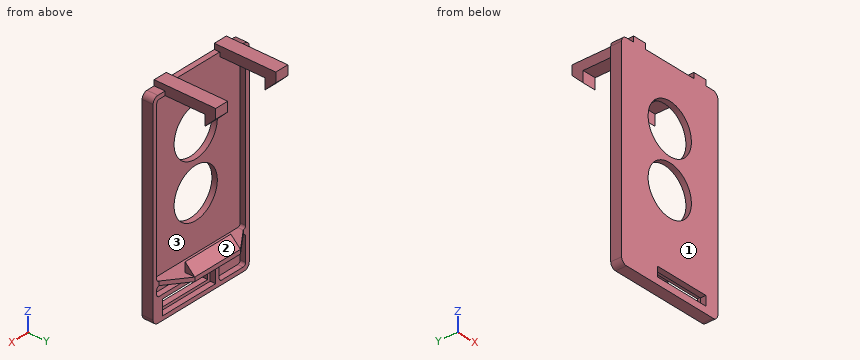
from build123d import *

# Parameters (mm, degrees)
BOSS_EXTRUDE1_DEPTH  = 1
PCB_HOLDER_52_R      = 4.5
BOSS_EXTRUDE2_DEPTH  = 1
BOSS_EXTRUDE3_DEPTH  = 2
PCB_HOLDER_57_W      = 17.5
PCB_HOLDER_57_H      = 0.75
BOSS_EXTRUDE7_DEPTH  = 5
SKETCH6_W            = 9.5
SKETCH6_H            = 1.75
BOSS_EXTRUDE9_DEPTH  = 1.75
CUT_EXTRUDE7_DEPTH   = 0.75
PCB_HOLDER_58_W      = 2.5
PCB_HOLDER_58_H      = 1
PCB_HOLDER_58_H_2    = 0.75
BOSS_EXTRUDE10_DEPTH = 11.25
SKETCH10_W           = 2.5
SKETCH10_H           = 2
BOSS_EXTRUDE11_DEPTH = 2
CUT_EXTRUDE8_DEPTH   = 15
CUT_EXTRUDE12_DEPTH  = 9.5
SKETCH12_W           = 11
SKETCH12_H           = 2.75
SKETCH12_W_2         = 10
SKETCH12_H_2         = 1.75
CUT_EXTRUDE15_DEPTH  = 1
SKETCH12_3_W         = 10
SKETCH12_3_H         = 1.75
CUT_EXTRUDE16_DEPTH  = 2


with BuildPart() as part:
    # PCB holder → Boss-Extrude1 (new body)
    with BuildSketch(Plane(origin=(0, 0, 0), x_dir=(1, 0, 0), z_dir=(0, 1, 0))):
        with BuildLine():
            Line((9, 21.5), (-9, 21.5))
            ThreePointArc((-9, 21.5), (-9.707106781, 21.207106781), (-10, 20.5))
            Line((-10, 20.5), (-10, -14.5))
            ThreePointArc((-10, -14.5), (-9.707106781, -15.207106781), (-9, -15.5))
            Line((-9, -15.5), (9, -15.5))
            ThreePointArc((9, -15.5), (9.707106781, -15.207106781), (10, -14.5))
            Line((10, -14.5), (10, 20.5))
            ThreePointArc((10, 20.5), (9.707106781, 21.207106781), (9, 21.5))
        make_face()
        with BuildLine():
            Line((9.25, 14.25), (9.25, -14.25))
            ThreePointArc((9.25, -14.25), (9.103553391, -14.603553391), (8.75, -14.75))
            Line((8.75, -14.75), (-8.75, -14.75))
            ThreePointArc((-8.75, -14.75), (-9.103553391, -14.603553391), (-9.25, -14.25))
            Line((-9.25, -14.25), (-9.25, 14.25))
            ThreePointArc((-9.25, 14.25), (-9.103553391, 14.603553391), (-8.75, 14.75))
            Line((-8.75, 14.75), (8.75, 14.75))
            ThreePointArc((8.75, 14.75), (9.103553391, 14.603553391), (9.25, 14.25))
        make_face(mode=Mode.SUBTRACT)
    extrude(amount=BOSS_EXTRUDE1_DEPTH)

    # PCB holder<52> → Boss-Extrude2 (add)
    with BuildSketch(Plane(origin=(0, 0, 0), x_dir=(1, 0, 0), z_dir=(0, 1, 0))):
        with BuildLine():
            Line((-9.25, 14.25), (-9.25, -14.25))
            ThreePointArc((-9.25, -14.25), (-9.103553391, -14.603553391), (-8.75, -14.75))
            Line((-8.75, -14.75), (8.75, -14.75))
            ThreePointArc((8.75, -14.75), (9.103553391, -14.603553391), (9.25, -14.25))
            Line((9.25, -14.25), (9.25, 14.25))
            ThreePointArc((9.25, 14.25), (9.103553391, 14.603553391), (8.75, 14.75))
            Line((8.75, 14.75), (-8.75, 14.75))
            ThreePointArc((-8.75, 14.75), (-9.103553391, 14.603553391), (-9.25, 14.25))
        make_face()
        with Locations(Location((0, -5, 0), (0, 0, 270))):
            Circle(PCB_HOLDER_52_R, mode=Mode.SUBTRACT)
        with Locations(Location((0, 5, 0), (0, 0, 270))):
            Circle(PCB_HOLDER_52_R, mode=Mode.SUBTRACT)
    extrude(amount=BOSS_EXTRUDE2_DEPTH)

    # PCB holder<55> → Boss-Extrude3 (add)
    with BuildSketch(Plane(origin=(0, 0, 0), x_dir=(1, 0, 0), z_dir=(0, 1, 0))):
        with BuildLine():
            Line((8.75, 15.5), (8.75, 14.75))
            ThreePointArc((8.75, 14.75), (9.103553391, 14.603553391), (9.25, 14.25))
            Line((9.25, 14.25), (9.25, -14.25))
            ThreePointArc((9.25, -14.25), (9.103553391, -14.603553391), (8.75, -14.75))
            Line((8.75, -14.75), (7.5, -14.75))
            Line((7.5, -14.75), (7.5, -15.5))
            Line((7.5, -15.5), (9, -15.5))
            ThreePointArc((9, -15.5), (9.707106781, -15.207106781), (10, -14.5))
            Line((10, -14.5), (10, 20.5))
            ThreePointArc((10, 20.5), (9.707106781, 21.207106781), (9, 21.5))
            Line((9, 21.5), (-9, 21.5))
            ThreePointArc((-9, 21.5), (-9.707106781, 21.207106781), (-10, 20.5))
            Line((-10, 20.5), (-10, -14.5))
            ThreePointArc((-10, -14.5), (-9.707106781, -15.207106781), (-9, -15.5))
            Line((-9, -15.5), (-7.5, -15.5))
            Line((-7.5, -15.5), (-7.5, -14.75))
            Line((-7.5, -14.75), (-8.75, -14.75))
            ThreePointArc((-8.75, -14.75), (-9.103553391, -14.603553391), (-9.25, -14.25))
            Line((-9.25, -14.25), (-9.25, 14.25))
            ThreePointArc((-9.25, 14.25), (-9.103553391, 14.603553391), (-8.75, 14.75))
            Line((-8.75, 14.75), (-8.75, 15.5))
            Line((-8.75, 15.5), (8.75, 15.5))
        make_face()
    extrude(amount=BOSS_EXTRUDE3_DEPTH)

    # PCB holder<57> → Boss-Extrude7 (add)
    with BuildSketch(Plane(origin=(0, 0, 0), x_dir=(1, 0, 0), z_dir=(0, 1, 0))):
        with Locations((0, 15.125)):
            Rectangle(PCB_HOLDER_57_W, PCB_HOLDER_57_H)
    extrude(amount=BOSS_EXTRUDE7_DEPTH)

    # Sketch6 → Boss-Extrude9 (add)
    with BuildSketch(Plane.XY.offset(-14.75)):
        with Locations((0, 4.125)):
            Rectangle(SKETCH6_W, SKETCH6_H)
    extrude(amount=BOSS_EXTRUDE9_DEPTH)

    # Sketch8 → Cut-Extrude7 (cut)
    with BuildSketch(Plane.XY.offset(-14.75)):
        Polygon((4.75, 5), (8.75, 2), (8.75, 5), align=None)
        Polygon((-4.75, 5), (-8.75, 2), (-8.75, 5), align=None)
    extrude(amount=-CUT_EXTRUDE7_DEPTH, mode=Mode.SUBTRACT)

    # PCB holder<58> → Boss-Extrude10 (add)
    with BuildSketch(Plane(origin=(0, 0, 0), x_dir=(1, 0, 0), z_dir=(0, 1, 0))):
        with Locations((-6.25, -16)):
            Rectangle(PCB_HOLDER_58_W, PCB_HOLDER_58_H)
        with Locations((-6.25, -15.125)):
            Rectangle(PCB_HOLDER_58_W, PCB_HOLDER_58_H_2)
        with Locations((6.25, -16)):
            Rectangle(PCB_HOLDER_58_W, PCB_HOLDER_58_H)
        with Locations((6.25, -15.125)):
            Rectangle(PCB_HOLDER_58_W, PCB_HOLDER_58_H_2)
    extrude(amount=BOSS_EXTRUDE10_DEPTH)

    # Sketch10 → Boss-Extrude11 (add)
    with BuildSketch(Plane(origin=(0, 0, 14.75), x_dir=(-1, 0, 0), z_dir=(0, 0, -1))):
        with Locations((-6.25, 10.25)):
            Rectangle(SKETCH10_W, SKETCH10_H)
        with Locations((6.25, 10.25)):
            Rectangle(SKETCH10_W, SKETCH10_H)
    extrude(amount=BOSS_EXTRUDE11_DEPTH)

    # Sketch11 → Cut-Extrude8 (cut)
    with BuildSketch(Plane(origin=(7.5, 0, 0), x_dir=(0, 0, -1), z_dir=(1, 0, 0))):
        Polygon((-14.75, 11.25), (-12.75, 9.25), (-12.75, 11.25), align=None)
    extrude(amount=-CUT_EXTRUDE8_DEPTH, mode=Mode.SUBTRACT)

    # Sketch7 → Cut-Extrude12 (cut)
    with BuildSketch(Plane(origin=(4.75, 0, 0), x_dir=(0, 0, -1), z_dir=(1, 0, 0))):
        Polygon((13, 3.25), (14.75, 5), (13, 5), align=None)
    extrude(amount=-CUT_EXTRUDE12_DEPTH, mode=Mode.SUBTRACT)

    # Sketch12 → Cut-Extrude15 (cut)
    # profile 1 of 2: a face of its own
    with BuildSketch(Plane(origin=(0, 2, 0), x_dir=(1, 0, 0), z_dir=(0, 1, 0))):
        with BuildLine():
            Line((9.25, 16), (9.25, 16.75))
            ThreePointArc((9.25, 16.75), (9.103553391, 17.103553391), (8.75, 17.25))
            Line((8.75, 17.25), (-3.25, 17.25))
            ThreePointArc((-3.25, 17.25), (-3.603553391, 17.396446609), (-3.75, 17.75))
            Line((-3.75, 17.75), (-3.75, 20.25))
            ThreePointArc((-3.75, 20.25), (-3.896446609, 20.603553391), (-4.25, 20.75))
            Line((-4.25, 20.75), (-8.75, 20.75))
            ThreePointArc((-8.75, 20.75), (-9.103553391, 20.603553391), (-9.25, 20.25))
            Line((-9.25, 20.25), (-9.25, 16))
            ThreePointArc((-9.25, 16), (-9.103553391, 15.646446609), (-8.75, 15.5))
            Line((-8.75, 15.5), (8.75, 15.5))
            ThreePointArc((8.75, 15.5), (9.103553391, 15.646446609), (9.25, 16))
        make_face()
    # profile 2 of 2: a face of its own
    with BuildSketch(Plane(origin=(0, 2, 0), x_dir=(1, 0, 0), z_dir=(0, 1, 0))):
        with Locations((2.5, 19.375)):
            Rectangle(SKETCH12_W, SKETCH12_H)
        with Locations((2.5, 19.375)):
            Rectangle(SKETCH12_W_2, SKETCH12_H_2, mode=Mode.SUBTRACT)
    extrude(amount=-CUT_EXTRUDE15_DEPTH, mode=Mode.SUBTRACT)

    # Sketch12<3> → Cut-Extrude16 (cut)
    with BuildSketch(Plane(origin=(0, 2, 0), x_dir=(1, 0, 0), z_dir=(0, 1, 0))):
        with Locations((2.5, 19.375)):
            Rectangle(SKETCH12_3_W, SKETCH12_3_H)
    extrude(amount=-CUT_EXTRUDE16_DEPTH, mode=Mode.SUBTRACT)


solid = part.part
Could you check a few things on this model? Use its own coordinates, in mm. Face numbers are marked on the shaded views. Give positions to 0.01 mm unless a question says otherwise; leave off trailing zeros. Write each loop counter-clockwise with the first axis right and the second up, starting at its lowest first coordinate (ties: lowest second). Pieces come first, ordered by that corner, then holes. Notation, with made-up numbers: (14, 30.25) - (55, 30.25) arc R23 cw to (55, 58.25) - close; hole circle Ø8 at (76, 4.5). An arc over 180 degrees is marked (long way). Use CSV: the item, a comma, the result in double quotes. Start each with the question number.
Item 1: I want a section at B-B, the plane z = 5. Please give me the cut outline in (x, y).
Item 2: If I drill on line 1 along X through (y, z) = (0.5, 5); line 2 along Z through (x, y) = (2.25, 1.25); line 3 along Y through (x, z) = (3.25, -0.5), over which ranges is the centre line in solid material (lowest first)?
Item 3: I want a section at A-A, the plane y = 10. Please give me the cut outline in (x, z), then the cut area to 3 significant figures.
Item 4: If we mould it in two halves opening along Z, with no side actions, what happens to the marked faces 1, 2 and 3? For each: pulls with the +Z half, pulls with the -Z half, needs draft (parallel to the pull), parting line crosses it, or undercut.
Item 5: I want a section at C-C, the plane x = 0. Please give me the cut outline in (y, z).
Item 6: I want a section at D-D, the plane y = 7.75. Please give me the cut outline in (x, z), then the cut area to 3 significant figures.
Item 7: I'm going to push flat-ended pins straight in: pin 1 (10 mm diameter, centred on x = -4, z = 2, fed in from -Y); pin 2 (1.9 mm diameter, centred on y = 7, z = 13.5, fed in from +X); pin 3 (1.2 mm diameter, centred on x = 2, y = 3.5, fed in from -Z); pin 4 (1.1 mm diameter, centred on y = 3.5, z = 14.5, fed in from +X). Where does each tip first touch, or does it pass through?
Findings:
1,outline,"(-10, 0) - (-4.5, 0) - (-4.5, 1) - (-9.25, 1) - (-9.25, 2) - (-10, 2) - close; (4.5, 0) - (10, 0) - (10, 2) - (9.25, 2) - (9.25, 1) - (4.5, 1) - close"
2,line 1,"x = -10 to -4.5, 4.5 to 10"
2,line 2,"z = -21.5 to -20.75, -18 to -17.25, -15.5 to -14.75"
2,line 3,"y = 0 to 1"
3,outline,"(-7.5, 13.5) - (-5, 13.5) - (-5, 16.5) - (-7.5, 16.5) - close; (5, 13.5) - (7.5, 13.5) - (7.5, 16.5) - (5, 16.5) - close"
3,area,"15.0 mm2"
4,face 1,"needs draft"
4,face 2,"pulls with the +Z half"
4,face 3,"undercut"
5,outline,"(0, -21.5) - (2, -21.5) - (2, -20.75) - (1, -20.75) - (1, -20.25) - (0, -20.25) - close; (0, -18.5) - (1, -18.5) - (1, -18) - (2, -18) - (2, -17.25) - (1, -17.25) - (1, -15.5) - (5, -15.5) - (5, -14.75) - (3.25, -13) - (3.25, -14.75) - (1, -14.75) - (1, -9.5) - (0, -9.5) - close; (0, -0.5) - (1, -0.5) - (1, 0.5) - (0, 0.5) - close; (0, 9.5) - (1, 9.5) - (1, 15.5) - (0, 15.5) - close"
6,outline,"(-7.5, 14.75) - (-5, 14.75) - (-5, 16.5) - (-7.5, 16.5) - close; (5, 14.75) - (7.5, 14.75) - (7.5, 16.5) - (5, 16.5) - close"
6,area,"8.75 mm2"
7,pin 1,"stops at y = 0"
7,pin 2,"passes through"
7,pin 3,"stops at z = -15.5"
7,pin 4,"stops at x = 7.5"
